The listing builds one solid part. Answer for the finished solid, in the listing's coordinates (mm). A direction names the side the tool comes from. Coordinates: 2 decimals unless noted, no trailing zeros. Order: outer loops, then holes, each group sorted by start corner. A loop starts at its lowest first (then second) coordinate and runs counter-clockwise, first axis right, second up.
from build123d import *

# Parameters (mm, degrees)
SKETCH154_R   = 1
SKETCH154_R_2 = 2.5
PAD078_DEPTH  = 1.6
SKETCH157_W   = 6
SKETCH157_H   = 6
PAD080_DEPTH  = 1.85


with BuildPart() as part:
    # Sketch154 → Pad078 (new body)
    with BuildSketch(Plane.XZ):
        Polygon((0.634909, -4.572), (-2.54, -1.397091), (-2.54, 21.208909), (-1.142757, 22.606152), (26.542463, 22.606152), (30.225783, 18.922833), (30.225783, -0.127127), (25.780909, -4.572), align=None)
        with Locations((0, 20.066152)):
            Circle(SKETCH154_R, mode=Mode.SUBTRACT)
        Circle(SKETCH154_R, mode=Mode.SUBTRACT)
        with Locations((20, 20.066152)):
            Circle(SKETCH154_R, mode=Mode.SUBTRACT)
        with Locations((20, 0.066152)):
            Circle(SKETCH154_R, mode=Mode.SUBTRACT)
        with Locations((10, 10)):
            Circle(SKETCH154_R_2, mode=Mode.SUBTRACT)
    extrude(amount=PAD078_DEPTH)

    # Sketch157 (on Face15 of Pad078) → Pad080 (join)
    with BuildSketch(Plane.XZ.offset(1.6)):
        with Locations((10, 10)):
            Rectangle(SKETCH157_W, SKETCH157_H)
    extrude(amount=PAD080_DEPTH)


with BuildPart() as part_1:
    # Body062 placement: moved
    add(part.part.moved(Location((5, 12, 12))))


solid = part_1.part
(1) The mould has two halves that part along Z. Classify faces 4 (the flat face through (19, 10.4, 21)), 5 (the flat face through (15, 10.4, 22)), 6 (the cylindrical face through (5, 11, 11)), 7 (the flat face through (15, 9, 19)): pulls with the +Z half, pulls with the -Z half, needs draft (parallel to the pull), parting line crosses it, or undercut.
(2) Find the intervals of material crossed by probe 1 along Z at (x, y) = (25, 11.6); probe 2 along Z at (x, y) = (15, 11.3); probe 3 along Y at (x, z) = (10, 11.75), in increasing order.
(3) Find section A-A on x = 25. Determine the outline of the cut face in (y, z), then the cut area to 3 significant figures.
(4) Find section B-B on z = 12.5. Determine the outline of the cut face in (x, y), then the cut area to 3 significant figures.
(5) Given pin 1 Ø2 at (y, z) = (9.5, 21.5) entering from -X; pin 2 Ø2 at (y, z) = (9, 24) entering from -X; pin 3 Ø1.5 at (x, y) = (15.5, 9.5) entering from +Z; pin 4 Ø2.5 at (x, z) = (15.5, 21) entering from +Y, each flat-ended and moving along its own axis, determine where each tip first touches the part or whether it passes through.
(6) A tool of negligible diameter and unlimited length cuts with its end or side. For faces 1 (the flat face through (18, 9, 22)), 2 (the flat face through (15, 9, 25)), 3 (the flat face through (12, 9, 22)), from which of +Z, -Z, +X, -X, +Y, -Y can it reach the whole face along a straight path? Write none if from no direction.
(7) Find section C-C on y = 10.75. Determine the outline of the cut face in (x, z), then the cut area to 3 significant figures.
(8) Find section D-D on z = 22. Determine the outline of the cut face in (x, y).
Resolved:
1. face 4: needs draft
1. face 5: undercut
1. face 6: undercut
1. face 7: pulls with the -Z half
2. probe 1: z = 7.43 to 11.07, 13.07 to 31.07, 33.07 to 34.61
2. probe 2: z = 7.43 to 19.5, 24.5 to 34.61
2. probe 3: y = 10.4 to 12
3. outline: (10.4, 7.43) - (12, 7.43) - (12, 11.07) - (10.4, 11.07) - close; (10.4, 13.07) - (12, 13.07) - (12, 31.07) - (10.4, 31.07) - close; (10.4, 33.07) - (12, 33.07) - (12, 34.61) - (10.4, 34.61) - close
3. area: 37.1 mm2
4. outline: (2.46, 10.4) - (4.13, 10.4) - (4.13, 12) - (2.46, 12) - close; (5.87, 10.4) - (24.1, 10.4) - (24.1, 12) - (5.87, 12) - close; (25.9, 10.4) - (35.23, 10.4) - (35.23, 12) - (25.9, 12) - close
4. area: 46.8 mm2
5. pin 1: stops at x = 2.46
5. pin 2: stops at x = 12
5. pin 3: stops at z = 25
5. pin 4: stops at y = 10.4
6. face 1: +Z, -Z, +X, -Y
6. face 2: +Z, +X, -X, -Y
6. face 3: +Z, -Z, -X, -Y
7. outline: (2.46, 10.6) - (5.63, 7.43) - (30.78, 7.43) - (35.23, 11.87) - (35.23, 30.92) - (31.54, 34.61) - (3.86, 34.61) - (2.46, 33.21) - close; hole circle Ø2 at (5, 12); hole circle Ø2 at (5, 32.07); hole circle Ø5 at (15, 22); hole circle Ø2 at (25, 12.07); hole circle Ø2 at (25, 32.07)
7. area: 836 mm2
8. outline: (2.46, 10.4) - (12, 10.4) - (12, 8.55) - (18, 8.55) - (18, 10.4) - (35.23, 10.4) - (35.23, 12) - (17.5, 12) - (17.5, 10.4) - (12.5, 10.4) - (12.5, 12) - (2.46, 12) - close
